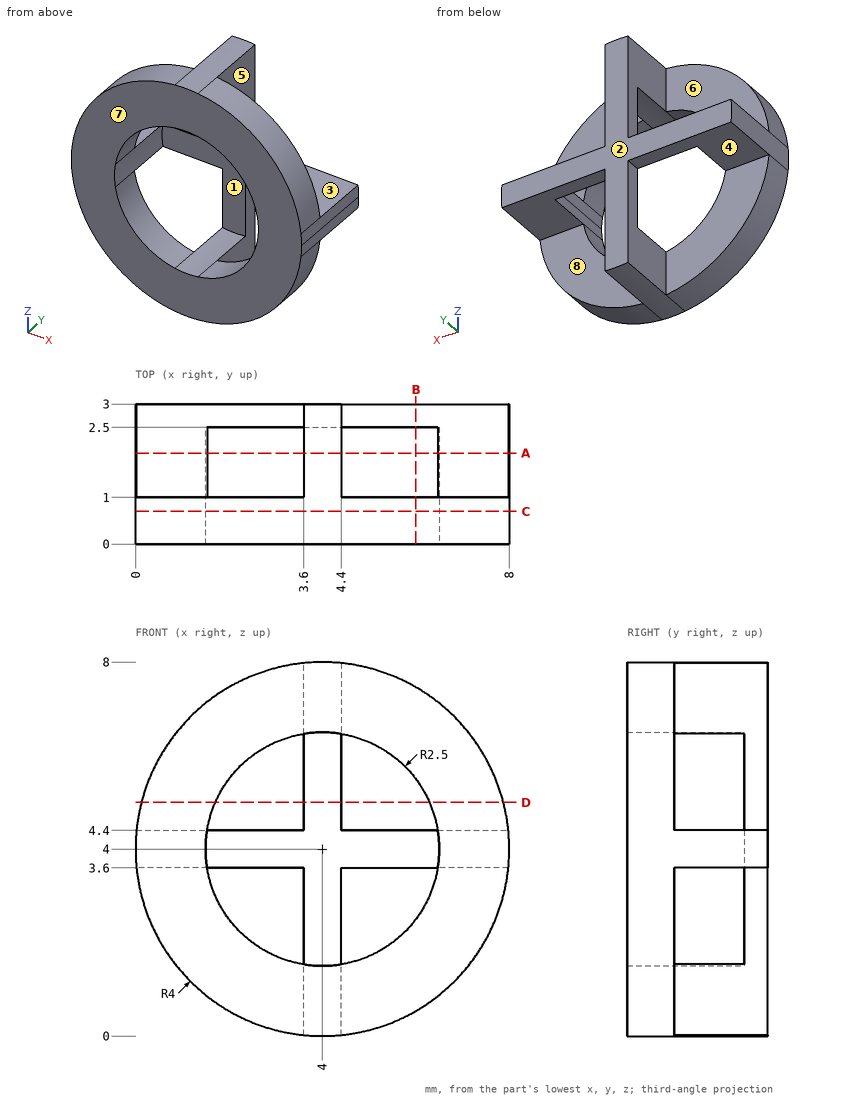
Check sheet for the drawn part. Datum: minimum x, y, z corner. Units: mm. A direction names the side the tool comes from. Coordinates: 2 decimals unless noted, no trailing zeros. Order: outer loops, then holes, each group sorted by start corner. A loop starts at its lowest first (then second) coordinate and runs counter-clockwise, first axis right, second up. Notation, with made-up numbers: M 85,-15 L 93,-15 A17 cw 93,-1 Z; hole C 23,5.25 d8. An arc over 180 degrees is marked long. One line per question, with ' | ' between items. Start each with the question number.
Item 1: Set-up check for the marked faces 4, 5, 6, 7 and 8: record each of +Z, -Z, +X, -X, +Y, -Y from which the full face is reachable in a straight line by a thin tool's end or side.
Item 2: Material ranges on L1, parallel to X at y = 2.8, z = 3; L2, parallel to Y at x = 7.25, z = 2.75, recorded low to high. Write a range as [from, to].
Item 3: Cross-section at D-D on z = 5. Enter the section's corners in (x, y), then the cut area to 3 significant figures.
Item 4: Cross-section at C-C on y = 0.7. Enter the section's corners in (x, z), then the cut area to 3 significant figures.
Item 5: Gauge pin test, flat ends, axial feed: pin 1 (1.8 mm diameter, centred on x = 2.5, z = 2.5, fed in from +Y); pin 2 (1.6 mm diameter, centred on y = 2.5, z = 1, fed in from +X); pin 3 (0.6 mm diameter, centred on x = 6, y = 1.5, fed in from -Z); pin 4 (1.6 mm diameter, centred on x = 1.5, y = 2, fed in from -Z). Record the tip position at first contact, or that the pin passes through.
Item 6: Draft check along Z on the marked faces 1, 2 and 3. Enter one of: pulls with the +Z half, pulls with the -Z half, needs draft (parallel to the pull), parting line crosses it, or undercut.
Item 7: Cross-section at A-A on y = 1.95. Enter the section's corners in (x, z), then the cut area to 3 significant figures.
Item 8: Cross-section at B-B on x = 6. Enter the section's corners in (y, z), then the cut area to 3 significant figures.
Findings:
1) face 4: -Z, -X, +Y | face 5: +Z, +X, +Y | face 6: +Z, -X, +Y | face 7: +Z, -Z, +X, -X, -Y | face 8: -Z, +X, +Y
2) L1: x = [3.6, 4.4] | L2: y = [0, 1]
3) outline: M 0.13,0 L 1.71,0 L 1.71,1 L 0.13,1 Z; M 3.6,2.5 L 4.4,2.5 L 4.4,3 L 3.6,3 Z; M 6.29,0 L 7.87,0 L 7.87,1 L 6.29,1 Z | area: 3.56 mm²
4) outline: C 4,4 d8; hole C 4,4 d5 | area: 30.6 mm²
5) pin 1: stops at y = 1 | pin 2: stops at x = 4.4 | pin 3: passes through | pin 4: stops at z = 3.6
6) face 1: undercut | face 2: needs draft | face 3: pulls with the +Z half
7) outline: M 0.02,3.6 L 1.53,3.6 A2.5 cw 1.53,4.4 L 0.02,4.4 A4 ccw Z; M 3.6,0.02 A4 ccw 4.4,0.02 L 4.4,1.53 A2.5 cw 3.6,1.53 Z; M 3.6,6.47 A2.5 cw 4.4,6.47 L 4.4,7.98 A4 ccw 3.6,7.98 Z; M 6.47,3.6 L 7.98,3.6 A4 ccw 7.98,4.4 L 6.47,4.4 A2.5 cw Z | area: 4.81 mm²
8) outline: M 0,0.54 L 1,0.54 L 1,2.5 L 0,2.5 Z; M 0,5.5 L 1,5.5 L 1,7.46 L 0,7.46 Z; M 2.5,3.6 L 3,3.6 L 3,4.4 L 2.5,4.4 Z | area: 4.33 mm²
